Geometry: final body of the model. Coordinates: model frame, mm. Face numbers are marked on the shaded views. A direction names the side the tool comes from. Coordinates: 2 decimals unless noted, no trailing zeros. Order: outer loops, then holes, each group sorted by start corner. A loop starts at its lowest first (then second) coordinate and runs counter-clockwise, first axis right, second up. Notation, with made-up numbers: (69, 55.5) -> (118, 55.5) arc R21 cw to (118, 76.5) -> close; hole circle Ø7 at (-3.5, -19). An arc over 180 degrees is marked (long way). Use one line per item in the form item = value.
```python
from build123d import *

# Parameters (mm, degrees)
BOSS_EXTRUDE1_DEPTH = 20
SHELL1_T            = -1.2


with BuildPart() as part:
    # Sketch2 → Boss-Extrude1 (new body)
    with BuildSketch(Plane(origin=(0, 0, 0), x_dir=(0, 0, -1), z_dir=(1, 0, 0))):
        Polygon((0, 0), (-22.067558379, 0), (28.64663303, 108.756934444), (232.463172314, 203.682917329), (232.463172314, 181.620135221), (43.694156178, 93.70242031), align=None)
    extrude(amount=BOSS_EXTRUDE1_DEPTH)

    # Shell1
    shell1_openings = [part.faces().sort_by_distance(p)[0] for p in [
        (10, 0, 11.03377919),
        (10, 192.651526275, -232.463172314),
    ]]
    offset(amount=SHELL1_T, openings=shell1_openings, kind=Kind.INTERSECTION)


solid = part.part
```
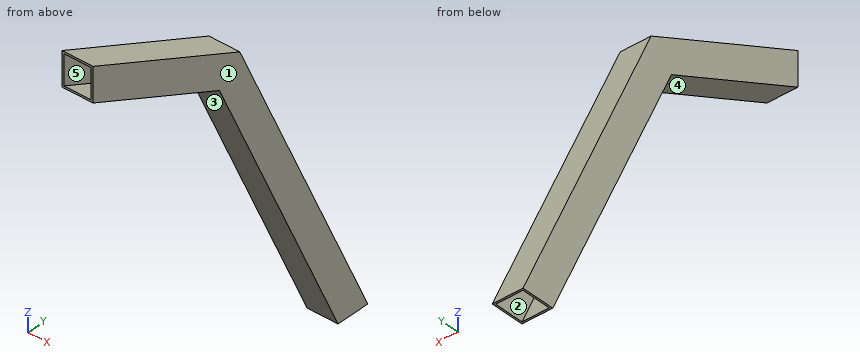
1) Contact query for flat-ended pins moving along their axis: P1, Ø6, axis at x = 14.5, z = -45.5, coming from the -Y side; P2, Ø8, axis at x = 11, z = -129, coming from the -Y side; P3, Ø6, axis at x = 3.5, y = 156.5, coming from the +Z side. Output: stop coordinate, or through.
Results found:
P1 = 91.14
P2 = 131.57
P3 = -124.71
2) Access query for the marked faces 4 and 5. Directions: +Z, -Z, +X, -X, +Y, -Y. A direction counts if a zero-diameter tool reaches every point of the face in a straight line with its end or side. Return the directions, or none.
Results found:
face_4 = -Z, +X, -X, -Y
face_5 = none
3) Pull-direction query (Y, two-part tool) for the marked faces 1, 2 and 3; classes: released by +Y, released by -Y, zero draft, split by the parting line, or undercut.
Results found:
face_1 = zero draft
face_2 = undercut
face_3 = released by -Y
4) Section C-C, the plane z = -99. Output: boundary loops of the cut face in (x, y), and give its area (3 significant figures).
Results found:
outline = (0, 119.46) -> (20, 119.46) -> (20, 141.52) -> (0, 141.52) -> close; hole (1.2, 120.78) -> (18.8, 120.78) -> (18.8, 140.2) -> (1.2, 140.2) -> close
area = 99.5 mm2
5) Section B-B, the plane y = 61. Output: boundary loops of the cut face in (x, z), and give its area (3 significant figures).
Results found:
outline = (0, -28.44) -> (20, -28.44) -> (20, -6.38) -> (0, -6.38) -> close; hole (1.2, -27.12) -> (18.8, -27.12) -> (18.8, -7.7) -> (1.2, -7.7) -> close
area = 99.6 mm2
6) Section A-A, the plane x = 13.25. Output: boundary loops of the cut face in (y, z).
Results found:
outline = (0, 0) -> (93.7, -43.69) -> (181.62, -232.46) -> (182.94, -232.46) -> (94.61, -42.79) -> (0, 1.32) -> close; (0, 20.74) -> (107.85, -29.55) -> (202.36, -232.46) -> (203.68, -232.46) -> (108.76, -28.65) -> (0, 22.07) -> close
7) Material intervals for probe 1 along X at (y, z) = (107.5, -37.5); probe 2 along Y at (x, z) = (3.75, -49); probe 3 along Z at (x, y) = (10, 67), sorted ascending. Write a range as from..to.
Results found:
probe_1 = 0..1.2, 18.8..20
probe_2 = 96.17..97.5, 116.91..118.24
probe_3 = -31.24..-29.92, -10.5..-9.18
